Verification items for the finished model (mm, model axes). Face numbers are marked on the shaded views. A direction names the side the tool comes from. Coordinates: 2 decimals unless noted, no trailing zeros. Write each loop counter-clockwise with the first axis right and the second up, starting at its lowest first coordinate (ties: lowest second). Pieces come first, ordered by that corner, then holes.
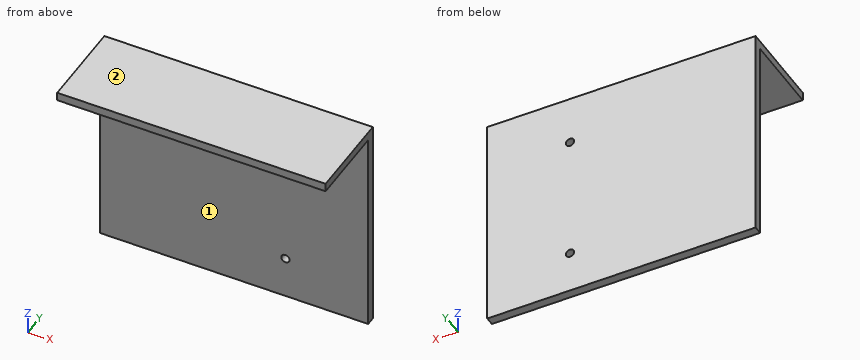
```python
from build123d import *

# Parameters (mm, degrees)
SKETCH1_W           = 94
SKETCH1_H           = 77
BOSS_EXTRUDE1_DEPTH = 3
SKETCH2_W           = 94
SKETCH2_H           = 3
BOSS_EXTRUDE2_DEPTH = 28.1
SKETCH3_R           = 1.45
CUT_EXTRUDE1_DEPTH  = 69.252912026
LPATTERN1_COUNT     = 2
LPATTERN1_PITCH     = 44.6


with BuildPart() as part:
    # Sketch1 → Boss-Extrude1 (new body)
    with BuildSketch(Plane(origin=(0, 0, 0), x_dir=(1, 0, 0), z_dir=(0, 1, 0))):
        Rectangle(SKETCH1_W, SKETCH1_H)
    extrude(amount=BOSS_EXTRUDE1_DEPTH)

    # Sketch2 → Boss-Extrude2 (add)
    with BuildSketch(Plane.XZ):
        with Locations((0, 37)):
            Rectangle(SKETCH2_W, SKETCH2_H)
    extrude(amount=BOSS_EXTRUDE2_DEPTH)

    # Sketch3 → Cut-Extrude1 (cut, through all)
    with BuildSketch(Plane(origin=(0, 3, 0), x_dir=(1, 0, 0), z_dir=(0, 1, 0))):
        with Locations(Location((18, 23.5, 0), (0, 0, 270))):
            Circle(SKETCH3_R)
    cut_extrude1 = extrude(amount=-CUT_EXTRUDE1_DEPTH, mode=Mode.SUBTRACT)

    # LPattern1: Cut-Extrude1 ×2
    with Locations(*[(0, 0, i * LPATTERN1_PITCH) for i in range(1, LPATTERN1_COUNT)]):
        add(cut_extrude1, mode=Mode.SUBTRACT)


solid = part.part
```
1. Sectioned sample at C-C, the plane y = -18. Record the boundary of the cut face in (x, z).
2. Tool access check on the marked faces 1 and 2. Record the directions out of +Z, -Z, +X, -X, +Y, -Y that give a thin tool (end or side, any length) a straight path to the whole face; none if there is none.
3. Gauge pin test, flat ends, axial feed: P1, Ø3, axis at x = 37, z = 28.5, coming from the -Y side; P2, Ø3, axis at x = 29.5, y = -18, coming from the -Z side; P3, Ø1.7, axis at x = 18, z = -23.5, coming from the +Y side. Record the tip position at first contact, or that the pin passes through.
4. Sectioned sample at D-D, the plane x = -18.5. Record the boundary of the cut face in (y, z), and give its area (3 significant figures).
5. Sectioned sample at B-B, the plane z = -23.5. Record the boundary of the cut face in (x, y).
6. Sectioned sample at A-A, the plane x = 18. Record the boundary of the cut face in (y, z), and give its area (3 significant figures).
7. Material ranges on L1, parallel to X at y = 1.25, z = 21.1; L2, parallel to Z at x = 37, y = -9.5; L3, parallel to Y at x = -2, z = -30.5, recorded low to high.
Outcome:
1. outline: (-47, 35.5) - (47, 35.5) - (47, 38.5) - (-47, 38.5) - close
2. face 1: -Z, +X, -X, -Y
2. face 2: +Z, +X, -X, +Y, -Y
3. P1: stops at y = 0
3. P2: stops at z = 35.5
3. P3: passes through
4. outline: (-28.1, 35.5) - (0, 35.5) - (0, -38.5) - (3, -38.5) - (3, 38.5) - (-28.1, 38.5) - close
4. area: 315 mm2
5. outline: (-47, 0) - (16.55, 0) - (16.55, 3) - (-47, 3) - close; (19.45, 0) - (47, 0) - (47, 3) - (19.45, 3) - close
6. outline: (-28.1, 35.5) - (0, 35.5) - (0, 22.55) - (3, 22.55) - (3, 38.5) - (-28.1, 38.5) - close; (0, -38.5) - (3, -38.5) - (3, -24.95) - (0, -24.95) - close; (0, -22.05) - (3, -22.05) - (3, 19.65) - (0, 19.65) - close
6. area: 298 mm2
7. L1: x = -47 to 16.55, 19.45 to 47
7. L2: z = 35.5 to 38.5
7. L3: y = 0 to 3
